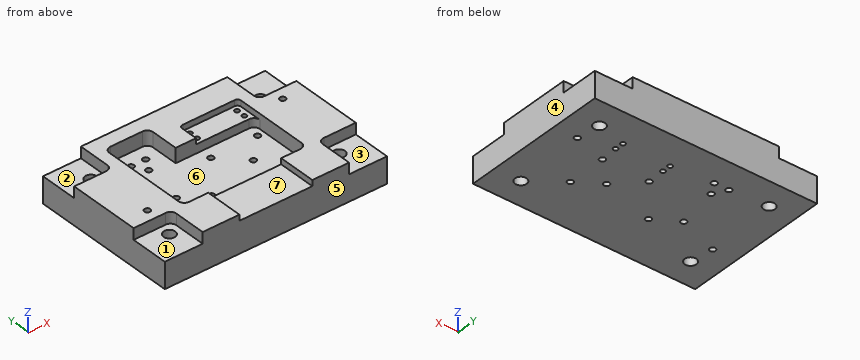
from build123d import *

# Parameters (mm, degrees)
CROQUIS1_W                      = 381
CROQUIS1_H                      = 254
SALIENTE_EXTRUIR1_DEPTH         = 63.5
CROQUIS2_W                      = 65
CROQUIS2_H                      = 65
CORTAR_EXTRUIR1_DEPTH           = 19
CORTAR_EXTRUIR2_DEPTH           = 10
CORTAR_EXTRUIR3_DEPTH           = 15
DI_METRO_DE_TALADRO_20_0_20_1_D = 20
DI_METRO_DE_TALADRO_10_0_10_1_D = 10
DI_METRO_DE_TALADRO_10_0_10_2_D = 10
DI_METRO_DE_TALADRO_8_0_8_1_D   = 8
REDONDEO1_R                     = 10
REDONDEO2_R                     = 6


with BuildPart() as part:
    # Croquis1 → Saliente-Extruir1 (new body)
    with BuildSketch(Plane.XY):
        Rectangle(CROQUIS1_W, CROQUIS1_H)
    extrude(amount=SALIENTE_EXTRUIR1_DEPTH)

    # Croquis2 → Cortar-Extruir1 (cut)
    with BuildSketch(Plane.XY.offset(63.5)):
        with Locations((-158, 94.5)):
            Rectangle(CROQUIS2_W, CROQUIS2_H)
        with Locations((-158, -94.5)):
            Rectangle(CROQUIS2_W, CROQUIS2_H)
        with Locations((158, -94.5)):
            Rectangle(CROQUIS2_W, CROQUIS2_H)
        with Locations((158, 94.5)):
            Rectangle(CROQUIS2_W, CROQUIS2_H)
    extrude(amount=-CORTAR_EXTRUIR1_DEPTH, mode=Mode.SUBTRACT)

    # Croquis3 → Cortar-Extruir2 (cut)
    with BuildSketch(Plane.XY.offset(63.5)):
        Polygon((62.5, -127), (62.5, -62), (105.5, -62), (105.5, 80), (4.5, 80), (4.5, 45), (-30.5, 45), (-30.5, 102), (-105.5, 102), (-105.5, -62), (-62.5, -62), (-62.5, -127), align=None)
    extrude(amount=-CORTAR_EXTRUIR2_DEPTH, mode=Mode.SUBTRACT)

    # Croquis4 → Cortar-Extruir3 (cut)
    with BuildSketch(Plane.XY.offset(53.5)):
        Polygon((105.5, -62), (105.5, 45), (-30.5, 45), (-30.5, 102), (-105.5, 102), (-105.5, -62), align=None)
    extrude(amount=-CORTAR_EXTRUIR3_DEPTH, mode=Mode.SUBTRACT)

    # Diámetro de taladro Ø20.0 (20)1 (through all)
    with Locations(Plane.XY.offset(44.5)):
        with Locations((-145.5, 82), (-145.5, -82), (145.5, -82), (145.5, 82)):
            Hole(DI_METRO_DE_TALADRO_20_0_20_1_D / 2)

    # Diámetro de taladro Ø10.0 (10)1 (through all)
    with Locations(Plane.XY.offset(38.5)):
        with Locations((-80.5, 77), (-55.5, 77), (-68, 55.349364905), (-80.5, -17), (-40.5, -42), (13.5, 25), (53.5, -15), (93.5, 25), (93.5, -42)):
            Hole(DI_METRO_DE_TALADRO_10_0_10_1_D / 2)

    # Diámetro de taladro Ø10.0 (10)2 (through all)
    with Locations(Plane.XY.offset(63.5)):
        with Locations((-150.5, -42), (150.5, 42)):
            Hole(DI_METRO_DE_TALADRO_10_0_10_2_D / 2)

    # Diámetro de taladro Ø8.0 (8)1 (through all)
    with Locations(Plane.XY.offset(53.5)):
        with Locations((14.5, 70), (95.5, 70), (95.5, 55), (14.5, 55)):
            Hole(DI_METRO_DE_TALADRO_8_0_8_1_D / 2)

    # Redondeo1
    redondeo1_edges = [part.edges().sort_by_distance(p)[0] for p in [
        (105.5, 45, 46),
        (125.5, 62, 54),
        (125.5, -62, 54),
        (-125.5, -62, 54),
        (-125.5, 62, 54),
        (-105.5, -62, 51),
        (-105.5, 102, 51),
        (-30.5, 102, 51),
        (105.5, -62, 51),
    ]]
    fillet(redondeo1_edges, radius=REDONDEO1_R)

    # Redondeo2
    redondeo2_edges = [part.edges().sort_by_distance(p)[0] for p in [
        (4.5, 80, 58.5),
        (105.5, 80, 58.5),
    ]]
    fillet(redondeo2_edges, radius=REDONDEO2_R)


solid = part.part
Can you work these out from the model? Positions are in its coordinate system, mm. Face numbers are marked on the shaded views. A direction names the side the tool comes from. Coordinates: 2 decimals unless noted, no trailing zeros. Write each loop counter-clockwise with the first axis right and the second up, starting at its lowest first coordinate (ties: lowest second). Pieces come first, ordered by that corner, then holes. Notation, with made-up numbers: (51, -20) -> (86, -20) arc R16 ccw to (86, -8) -> close; hole circle Ø8 at (-21, 42.25). An arc over 180 degrees is marked (long way). Write each question's results on one line, items separated by ' | '. Start each with the question number.
Q1. If I drill on probe 1 along Y at (x, z) = (-80.5, 24); probe 2 along Y at (x, z) = (13.5, 15.5); probe 3 along Y at (x, z) = (95.5, 15.5), over which ranges is the centre line in solid material (lowest first)?
Q2. Imagine slicing it at A-A (x = -55.5). Write out the boundary of the cut face in (y, z).
Q3. On a 3-axis mill with a long thin cutter (end or side, diameter ignored), from which of +Z, -Z, +X, -X, +Y, -Y can I reach the whole of each face in a straight line? I mean the marked faces 1, 2 and 3. Say none if no direction works.
Q4. Imagine slicing it at B-B (y = -82). Write out the boundary of the cut face in (x, z), then the cut area to 3 significant figures.
Q5. Imagine slicing it at C-C (y = -42). Write out the boundary of the cut face in (x, z), then the cut area to 3 significant figures.
Q6. I'm going to push flat-ended pins straight in: pin 1 (1.5 mm diameter, centred on x = 74.5, y = -95, fed in from -Z); pin 2 (3 mm diameter, centred on y = -104.5, z = 57.5, fed in from +X); pin 3 (5.5 mm diameter, centred on y = 93, z = 55, fed in from -X); pin 4 (8 mm diameter, centred on x = 93.5, y = -42, fed in from +Z). Where does each tip first touch, or does it pass through?
Q7. Imagine slicing it at D-D (z = 24). State how many separate pieces and enclosed holes the cut face has, then the cut area to 3 significant figures.
Q8. We'd pull the mould along X, two halves only. Please class the marked faces 4, 5, 6 and 7: +X half, -X half, draft (parallel to the pull), parting line (faces both ways), or undercut.
Taken from the geometry:
1) probe 1: y = -127 to -22, -12 to 72, 82 to 127 | probe 2: y = -127 to 20, 30 to 51.13, 58.87 to 66.13, 73.87 to 127 | probe 3: y = -127 to -46.58, -37.42 to 20.42, 29.58 to 51, 59 to 66, 74 to 127
2) outline: (-127, 0) -> (72, 0) -> (72, 38.5) -> (-62, 38.5) -> (-62, 53.5) -> (-127, 53.5) -> close; (82, 0) -> (127, 0) -> (127, 63.5) -> (102, 63.5) -> (102, 38.5) -> (82, 38.5) -> close
3) face 1: +Z, -X, -Y | face 2: +Z, -X, +Y | face 3: +Z, +X, -Y
4) outline: (-190.5, 0) -> (-155.5, 0) -> (-155.5, 44.5) -> (-190.5, 44.5) -> close; (-135.5, 0) -> (135.5, 0) -> (135.5, 44.5) -> (125.5, 44.5) -> (125.5, 63.5) -> (62.5, 63.5) -> (62.5, 53.5) -> (-62.5, 53.5) -> (-62.5, 63.5) -> (-125.5, 63.5) -> (-125.5, 44.5) -> (-135.5, 44.5) -> close; (155.5, 0) -> (190.5, 0) -> (190.5, 44.5) -> (155.5, 44.5) -> close | area: 18,700 mm^2
5) outline: (-190.5, 0) -> (-155.5, 0) -> (-155.5, 63.5) -> (-190.5, 63.5) -> close; (-145.5, 0) -> (-45.5, 0) -> (-45.5, 38.5) -> (-105.5, 38.5) -> (-105.5, 63.5) -> (-145.5, 63.5) -> close; (-35.5, 0) -> (88.5, 0) -> (88.5, 38.5) -> (-35.5, 38.5) -> close; (98.5, 0) -> (190.5, 0) -> (190.5, 63.5) -> (105.5, 63.5) -> (105.5, 38.5) -> (98.5, 38.5) -> close | area: 17,500 mm^2
6) pin 1: stops at z = 0 | pin 2: stops at x = 125.5 | pin 3: stops at x = -125.5 | pin 4: passes through
7) separate pieces: 1 | enclosed holes: 19 | area: 94,500 mm^2
8) face 4: +X half | face 5: draft | face 6: undercut | face 7: undercut
